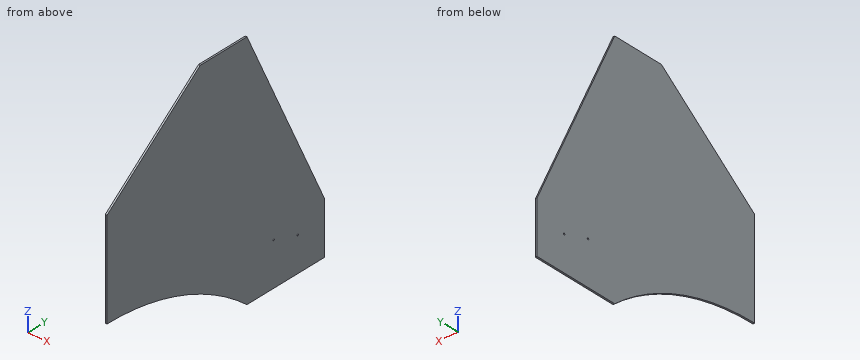
Autodesk Inventor part; units mm, degrees
ref_plane "YZ Plane" through (0, 0, 0) normal (1, 0, 0) x (0, 1, 0)
ref_plane "XZ Plane" through (0, 0, 0) normal (0, 1, 0) x (-1, 0, 0)
ref_plane "XY Plane" through (0, 0, 0) normal (0, 0, 1) x (1, 0, 0)
sketch "スケッチ1" plane through (0, 0, 0) normal (1, 0, 0) x (0, 1, 0)
  line L0 (-700, 170) -> (-700, 450)
  line L1 (-700, 450) -> (-400, 690)
  line L2 (-400, 690) -> (-250, 690)
  line L3 (-250, 690) -> (0, 150)
  line L4 (0, 150) -> (0, 0)
  line L5 (0, 0) -> (-250, 0)
  arc A0 (-250, 0) -> (-700, 170) centre (-700, -510.5882) ccw
  dimension "d0" = 690
  dimension "d1" = 280
  dimension "d2" = 240
  dimension "d3" = 300
  dimension "d4" = 150
  dimension "d5" = 700
  dimension "d6" = 250
  dimension "d7" = 150
extrude "押し出し1" add sketch "スケッチ1" along normal blind 5
sketch "スケッチ2" plane through (5, 0, 0) normal (1, 0, 0) x (0, 0, -1)
  circle A0 centre (-100, -87) radius 2.5
  line L0 (0, 0) -> (-150, 0)
  line L1 (0, -250) -> (0, 0)
  circle A1 centre (-125, -164) radius 2.5
  dimension "d10" = 87
  dimension "d11" = 100
  dimension "d12" = 5
  dimension "d13" = 164
  dimension "d14" = 125
  dimension "d15" = 5
extrude "押し出し2" cut sketch "スケッチ2" against normal through all
properties part number "end_plate" material "CFRP"
Can you work these out from the model? Positions are in its coordinate system, mm. Round coordinates to 2 decimals unless told otherwise and drop trailing zeros. Loops run counter-clockwise (first coordinate to the right, second up) from the corner with the lowest first, then second, coordinate; pieces in that order, holes last. Notation, with made-up numbers: M 6.5,77.5 L 32.5,77.5 A34 cw 32.5,113.5 Z; hole C -28.5,11.25 d6. An arc over 180 degrees is marked long. Answer as a JSON object with one key per item and string values. Group by question number.
Q1. Imagine slicing it at B-B, the plane y = -176.5. Please give me the cut outline in (x, z).
Q2. Please list where these lines run through material, in increasing order: L1, parallel to Z at x = 2.45, y = -164; L2, parallel to Y at x = 3.45, z = 100; L3, parallel to Z at x = 0.25, y = -555.
Q3. Imagine slicing it at A-A, the plane x = 1.5. Please give me the cut outline in (y, z).
Q4. Imagine slicing it at C-C, the plane z = 335.5. Please give me the cut outline in (x, y).
Findings:
{
 "1": {"outline": "M 0,0 L 5,0 L 5,531.24 L 0,531.24 Z"},
 "2": {"L1": "z = 0 to 122.5, 127.5 to 504.24", "L2": "y = -399.36 to -89.5, -84.5 to 0", "L3": "z = 154.37 to 566"},
 "3": {"outline": "M -700,170 A680.59 cw -250,0 L 0,0 L 0,150 L -250,690 L -400,690 L -700,450 Z; hole C -164,125 d5; hole C -87,100 d5"},
 "4": {"outline": "M 0,-700 L 5,-700 L 5,-85.88 L 0,-85.88 Z"}
}
